```python
from build123d import *

# Parameters (mm, degrees)
BOSS_EXTRU_1_DEPTH      = 6
ENL_V_MAT_EXTRU_1_REACH = 272.483
ESQUISSE2_R             = 2.75


with BuildPart() as part:
    # Esquisse1 → Boss.-Extru.1 (new body)
    with BuildSketch(Plane(origin=(0, 0, 0), x_dir=(1, 0, 0), z_dir=(0, 1, 0))):
        Polygon((-37.5, 194.855715851), (37.5, 194.855715851), (187.5, -64.951905284), (150, -129.903810568), (-150, -129.903810568), (-187.5, -64.951905284), align=None)
    extrude(amount=BOSS_EXTRU_1_DEPTH)

    # Esquisse2 → Enlèv. mat.-Extru.1 (cut, up to next)
    with BuildSketch(Plane(origin=(0, 6, 0), x_dir=(1, 0, 0), z_dir=(0, 1, 0)), mode=Mode.PRIVATE) as enl_v_mat_extru_1_sk1:
        with Locations(Location((0, 159.641425484, 0), (0, 0, 270))):
            Circle(ESQUISSE2_R)
    enl_v_mat_extru_1_tool1 = extrude(enl_v_mat_extru_1_sk1.sketch, amount=-ENL_V_MAT_EXTRU_1_REACH, mode=Mode.PRIVATE) & part.part
    # Esquisse2 → Enlèv. mat.-Extru.1 (cut, up to next)
    with BuildSketch(Plane(origin=(0, 6, 0), x_dir=(1, 0, 0), z_dir=(0, 1, 0)), mode=Mode.PRIVATE) as enl_v_mat_extru_1_sk2:
        with Locations(Location((-138.253529965, -79.820712742, 0), (0, 0, 270))):
            Circle(ESQUISSE2_R)
    enl_v_mat_extru_1_tool2 = extrude(enl_v_mat_extru_1_sk2.sketch, amount=-ENL_V_MAT_EXTRU_1_REACH, mode=Mode.PRIVATE) & part.part
    # Esquisse2 → Enlèv. mat.-Extru.1 (cut, up to next)
    with BuildSketch(Plane(origin=(0, 6, 0), x_dir=(1, 0, 0), z_dir=(0, 1, 0)), mode=Mode.PRIVATE) as enl_v_mat_extru_1_sk3:
        with Locations(Location((138.253529965, -79.820712742, 0), (0, 0, 270))):
            Circle(ESQUISSE2_R)
    enl_v_mat_extru_1_tool3 = extrude(enl_v_mat_extru_1_sk3.sketch, amount=-ENL_V_MAT_EXTRU_1_REACH, mode=Mode.PRIVATE) & part.part
    add(enl_v_mat_extru_1_tool1.solids().sort_by_distance((0, 6, -159.641425))[0], mode=Mode.SUBTRACT)
    add(enl_v_mat_extru_1_tool2.solids().sort_by_distance((-138.25353, 6, 79.820713))[0], mode=Mode.SUBTRACT)
    add(enl_v_mat_extru_1_tool3.solids().sort_by_distance((138.25353, 6, 79.820713))[0], mode=Mode.SUBTRACT)


solid = part.part
```
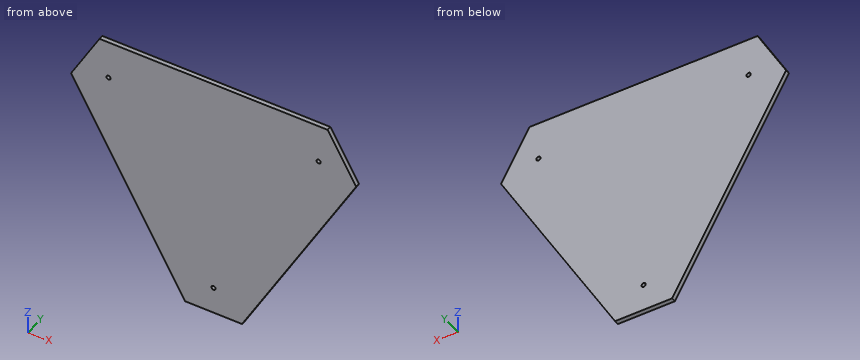
Can you work these out from the model? Positions are in its coordinate system, mm. Coordinates: 2 decimals unless noted, no trailing zeros. Order: outer loops, then holes, each group sorted by start corner. A loop starts at its lowest first (then second) coordinate and runs counter-clockwise, first axis right, second up. Notation, with made-up numbers: (74.25, -20.5) - (117.25, -20.5) arc R14 cw to (117.25, -16.5) - close; hole circle Ø7 at (5, -1). An arc over 180 degrees is marked (long way). Answer in a Markdown table with one row per item.
1. Suppose I cut it at C-C (x = -72). Please give me the cut outline in (y, z), and give its area (3 significant figures).
Reply:
| item | result |
|---|---|
| outline | (0, -135.1) - (6, -135.1) - (6, 129.9) - (0, 129.9) - close |
| area | 1,590 mm^2 |
2. If I drill on line 1 along Z through (x, y) = (-76, 5.65); line 2 along X through (y, z) = (4.3, -146); line 3 along X through (y, z) = (2.3, -106), over which ranges is the centre line in solid material (lowest first)?
Reply:
| item | result |
|---|---|
| line 1 | z = -128.17 to 129.9 |
| line 2 | x = -65.71 to 65.71 |
| line 3 | x = -88.8 to 88.8 |
3. Suppose I cut it at B-B (z = -32.5). Please give me the cut outline in (x, y).
Reply:
| item | result |
|---|---|
| outline | (-131.24, 0) - (131.24, 0) - (131.24, 6) - (-131.24, 6) - close |
4. Suppose I cut it at A-A (y = 2.7). Please give me the cut outline in (x, z), and give its area (3 significant figures).
Reply:
| item | result |
|---|---|
| outline | (-187.5, 64.95) - (-37.5, -194.86) - (37.5, -194.86) - (187.5, 64.95) - (150, 129.9) - (-150, 129.9) - close; hole circle Ø5.5 at (-138.25, 79.82); hole circle Ø5.5 at (0, -159.64); hole circle Ø5.5 at (138.25, 79.82) |
| area | 80,300 mm^2 |
5. For pin 1 (2 mm diameter, centred on y = 2, z = -26.5, fed in from -X); pin 2 (1 mm diameter, centred on x = 40.5, y = 5, fed in from -Z); pin 3 (1.5 mm diameter, centred on y = 1, z = -144.5, fed in from +X), each with a flat end and sliding along its axis, tell me the tip position at first contact or that it passes through.
Reply:
| item | result |
|---|---|
| pin 1 | stops at x = -135.28 |
| pin 2 | stops at z = -190.53 |
| pin 3 | stops at x = 67.01 |
